```python
from build123d import *

# Parameters (mm, degrees)
F0_R           = 12.7
F1_DEPTH       = 711.2
F3_DEPTH       = 19.05
F4_R           = 2.54
F7_DEPTH       = 45.72
F7_DEPTH_BACK  = 25.4
F9_DEPTH       = 25.4
F9_DEPTH_BACK  = 25.4
F10_R          = 3.175
F11_DEPTH      = 25.4
F11_DEPTH_BACK = 25.4


with BuildPart() as f1:
    # F0 (on Right) → F1 (new body)
    with BuildSketch(Plane.YZ):
        Circle(F0_R)
    extrude(amount=F1_DEPTH)

    # F2 (on Front) → F3 (join)
    with BuildSketch(Plane.XZ):
        with BuildLine():
            ThreePointArc((9.525, 0), (12.7, -3.175), (15.875, 0))
            ThreePointArc((15.875, 0), (12.7, 3.175), (9.525, 0))
        make_face()
    extrude(amount=F3_DEPTH)

    # F4
    f4_edges = [f1.edges().sort_by_distance(p)[0] for p in [
        (0, -12.7, 0),
        (711.2, -12.7, 0),
    ]]
    fillet(f4_edges, radius=F4_R)

    # F6 (on offset) → F7 (cut, two sides)
    with BuildSketch(Plane.XZ.offset(-6.35)) as f7_sk:
        with BuildLine():
            ThreePointArc((15.875, 0), (12.7, 3.175), (9.525, 0))
            Line((9.525, 0), (12.7, 0))
            Line((12.7, 0), (15.875, 0))
        make_face()
        with BuildLine():
            ThreePointArc((701.675, 0), (698.5, 3.175), (695.325, 0))
            ThreePointArc((695.325, 0), (698.5, -3.175), (701.675, 0))
        make_face()
        with BuildLine():
            Line((12.7, 0), (9.525, 0))
            ThreePointArc((9.525, 0), (12.7, -3.175), (15.875, 0))
            Line((15.875, 0), (12.7, 0))
        make_face()
    extrude(amount=-F7_DEPTH, mode=Mode.SUBTRACT)
    extrude(f7_sk.sketch, amount=F7_DEPTH_BACK, mode=Mode.SUBTRACT)

    # F8 (on Front) → F9 (cut, two sides)
    with BuildSketch(Plane.XZ) as f9_sk:
        with BuildLine():
            ThreePointArc((136.525, 0), (139.7, -3.175), (142.875, 0))
            ThreePointArc((142.875, 0), (139.7, 3.175), (136.525, 0))
        make_face()
    extrude(amount=-F9_DEPTH, mode=Mode.SUBTRACT)
    extrude(f9_sk.sketch, amount=F9_DEPTH_BACK, mode=Mode.SUBTRACT)

    # F10 (on Top) → F11 (cut, two sides)
    with BuildSketch(Plane.XY) as f11_sk:
        with BuildLine():
            ThreePointArc((22.225, 0), (25.4, -3.175), (28.575, 0))
            ThreePointArc((28.575, 0), (25.4, 3.175), (22.225, 0))
        make_face()
        with Locations((685.8, 0)):
            Circle(F10_R)
    extrude(amount=-F11_DEPTH, mode=Mode.SUBTRACT)
    extrude(f11_sk.sketch, amount=F11_DEPTH_BACK, mode=Mode.SUBTRACT)


solid = f1.part
```
Verification items for the finished model (mm, model axes). Coordinates: 2 decimals unless noted, no trailing zeros. Loops run counter-clockwise (first coordinate to the right, second up) from the corner with the lowest first, then second, coordinate; pieces in that order, holes last. Notation, with made-up numbers: (-21.5, -3) - (32.5, -3) arc R30 cw to (32.5, 30) - close; hole circle Ø1 at (29.5, -25). An arc over 180 degrees is marked (long way). Put each result on its own line as item: value.
Item 1: Section check A-A (x = 652.5). Enter the section's corners in (y, z), then the cut area to 3 significant figures.
Conclusion:
outline: circle Ø25.4 at (0, 0)
area: 507 mm2
Item 2: Scan lines: line 1 along X through (y, z) = (0.5, 6.5); line 2 along X through (y, z) = (5, -2); line 3 along X through (y, z) = (-10.5, -2.5). Record each from-to range of solid material in increasing order.
Conclusion:
line 1: x = 0 to 22.26, 28.54 to 682.66, 688.94 to 711.2
line 2: x = 0 to 10.23, 15.17 to 137.23, 142.17 to 696.03, 700.97 to 711.2
line 3: x = 0.08 to 10.74, 14.66 to 137.74, 141.66 to 696.54, 700.46 to 711.12
Item 3: Gauge pin test, flat ends, axial feed: pin 1 Ø12 at (x, z) = (178.5, -3) entering from -Y; pin 2 Ø2 at (x, z) = (371.5, -2) entering from +Y; pin 3 Ø5 at (x, y) = (201, -5.5) entering from +Z; pin 4 Ø6 at (x, y) = (404, -9.5) entering from -Z. Record the tip position at first contact, or that the pin passes through.
Conclusion:
pin 1: stops at y = -12.7
pin 2: stops at y = 12.66
pin 3: stops at z = 12.34
pin 4: stops at z = -10.91
Item 4: Draft check along Z on faces 1 (the face through (711.2, 0, 0)), 2 (the face through (350.66, -2.75, -12.4)). Enter one of: pulls with the +Z half, pulls with the -Z half, needs draft (parallel to the pull), parting line crosses it, or undercut.
Conclusion:
face 1: needs draft
face 2: parting line crosses it
